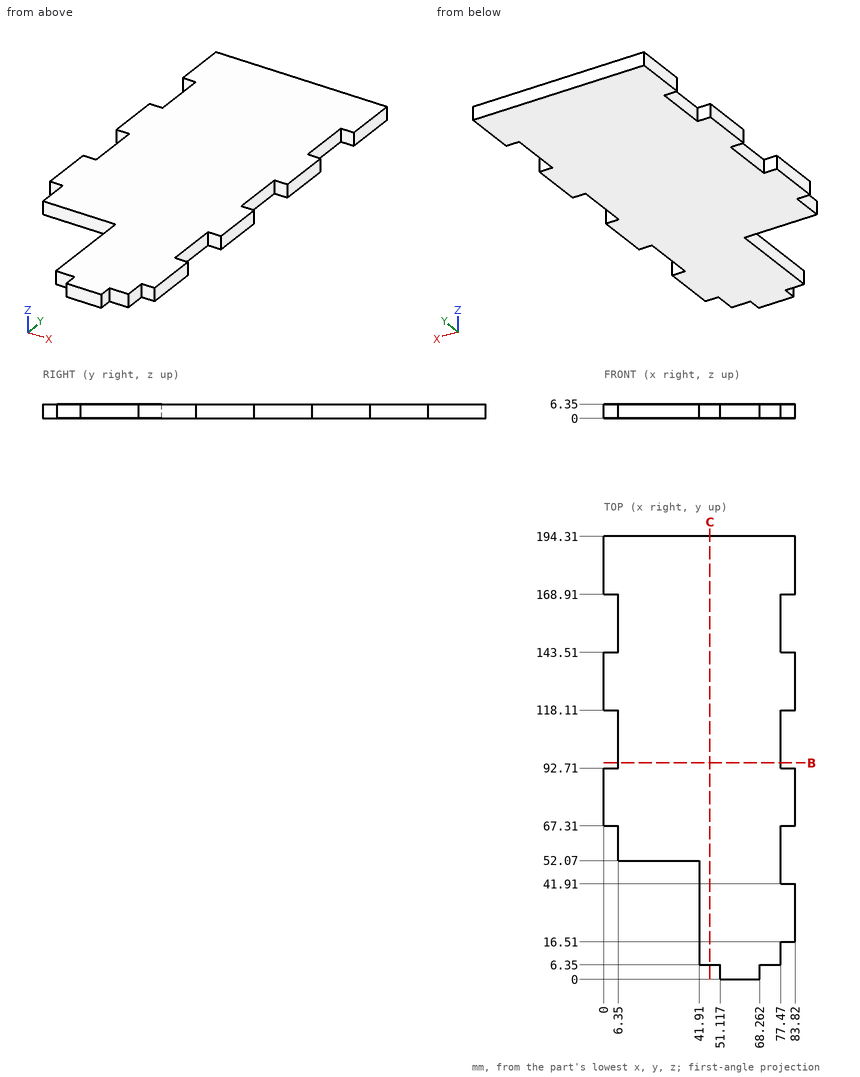
Verification items for this drawing (mm, ordinates from the low corner). Coordinates: 2 decimals unless noted, no trailing zeros. Order: outer loops, then holes, each group sorted by start corner. A loop starts at its lowest first (then second) coordinate and runs counter-clockwise, first axis right, second up. Notation, with made-up numbers: M -30,-40 L -3,-40 A11 ccw -3,-33 Z; hole C 73.5,71.25 d1. An arc over 180 degrees is marked long. One line per item, written item: value. Start each with the question number.
Item 1: Depth check by flat-ended pin: P1, Ø1.9, axis at y = 3.5, z = 1.5, coming from the +X side; P2, Ø1.9, axis at y = 152, z = 4.5, coming from the +X side; P3, Ø1.9, axis at y = 61.5, z = 4, coming from the -X side; P4, Ø3, axis at x = 43.5, y = 36.5, coming from the -Z side. Enter the tip coordinate at first touch or a pass-through.
Item 2: Thickness scan on probe 1 along Y at (x, z) = (48, 5.5); probe 2 along X at (y, z) = (50, 1); probe 3 along X at (y, z) = (157.5, 5). Record the ranges inside material, lowest first.
Item 3: Sectioned sample at B-B on y = 95. Record the cut outline in (x, z).
Item 4: Sectioned sample at C-C on x = 46.5. Record the cut outline in (y, z).
Calculated:
1. P1: x = 68.26
1. P2: x = 77.47
1. P3: x = 6.35
1. P4: z = 0
2. probe 1: 6.35 to 194.31
2. probe 2: 41.91 to 77.47
2. probe 3: 6.35 to 77.47
3. outline: M 6.35,0 L 77.47,0 L 77.47,6.35 L 6.35,6.35 Z
4. outline: M 6.35,0 L 194.31,0 L 194.31,6.35 L 6.35,6.35 Z
